```python
from build123d import *

# Parameters (mm, degrees)
F0_W     = 520.7
F0_H     = 457.2
F1_DEPTH = 36.5125
F2_R     = 203.2
F3_R     = 69.85
F4_R     = 22.225
F6_DEPTH = 222.25
F6_TAPER = -1
F8_ANGLE = 180


# Not quite as in the source:
# - a feature names something its author has since deleted; it is built from what else it names


with BuildPart() as f1:
    # F0 (on Top) → F1 (new body)
    with BuildSketch(Plane.XY):
        Rectangle(F0_W, F0_H)
    extrude(amount=F1_DEPTH)

    # F2
    f2_edges = [f1.edges().sort_by_distance(p)[0] for p in [
        (-260.35, -228.6, 18.25625),
        (260.35, -228.6, 18.25625),
    ]]
    fillet(f2_edges, radius=F2_R)

    # F3
    f3_edges = [f1.edges().sort_by_distance(p)[0] for p in [
        (260.35, 228.6, 18.25625),
        (-260.35, 228.6, 18.25625),
    ]]
    fillet(f3_edges, radius=F3_R)

    # F4
    f4_edges = [f1.edges().sort_by_distance(p)[0] for p in [
        (0, 228.6, 36.5125),
    ]]
    fillet(f4_edges, radius=F4_R)

    # F5 (on face) → F6 (cut)
    with BuildSketch(Plane(origin=(0, 228.6, 0), x_dir=(-1, 0, 0), z_dir=(0, 1, 0))):
        with BuildLine():
            Line((0, 181.2540946981), (-105.1541626057, 217.9785540242))
            ThreePointArc((-105.1541626057, 217.9785540242), (-243.9245415433, 129.7884295676), (-126.0241182101, 15.1838646496))
            Line((-126.0241182101, 15.1838646496), (0, 31.7752545682))
            Line((0, 31.7752545682), (126.0241182101, 15.1838646496))
            ThreePointArc((126.0241182101, 15.1838646496), (243.9245415433, 129.7884295676), (105.1541626057, 217.9785540242))
            Line((105.1541626057, 217.9785540242), (0, 181.2540946981))
        make_face()
    extrude(amount=-F6_DEPTH, taper=F6_TAPER, mode=Mode.SUBTRACT)

    # F7 (on face) → F8 (revolve, cut)
    with BuildSketch(Plane(origin=(0, 6.35, 0), x_dir=(-1, 0, 0), z_dir=(0, 1, 0))):
        with BuildLine():
            Line((0, 36.5125), (-210.3489459995, 36.5125))
            ThreePointArc((-210.3489459995, 36.5125), (-170.6122176221, 14.8981545045), (-125.5177564428, 11.3376651729))
            Line((-125.5177564428, 11.3376651729), (0, 27.8623913002))
            Line((0, 27.8623913002), (0, 36.5125))
        make_face()
    revolve(axis=Axis((0, 6.35, 32.1874456501), (0, 0, -1)), revolution_arc=F8_ANGLE, mode=Mode.SUBTRACT)


solid = f1.part
```
Work out the finished part from the listing and answer in its coordinate system (mm). A direction names the side the tool comes from. Round coordinates to 2 decimals unless told otherwise and drop trailing zeros. Return JSON: item names as keys, results as strings. Group by question number.
Q1. Find the intervals of material crossed by L1, parallel to Z at x = -236.5, y = -54.5; L2, parallel to X at y = 156, z = 31.5; L3, parallel to X at y = -129.5, z = 34, in increasing order.
Q2. Each of these flat-tipped pins is pushed along its axis until it touches: pin 1 Ø12 at (y, z) = (149, 23.5) entering from -X; pin 2 Ø4 at (x, z) = (-10.5, 27) entering from -Y; pin 3 Ø6 at (x, z) = (-67, 19.5) entering from -Y. Where does it stop, or does it pass through?
Q3. For faces 5 (the conical face through (170.668, 115.919, 16.912)), 6 (the flat face through (260.35, 65, 7)), determine the directions among +Z, -Z, +X, -X, +Y, -Y from which every point of the face is accessible in a straight line to the end or side of a thin tool.
Q4. The mould has two halves that part along Y. Classify faces 1 (the conical face through (-169.467, 115.919, 16.555)), 2 (the flat face through (-54, -198, 36.512)), 3 (the cylindrical face through (239.345, 208.681, 7.244)), 4 (the cylindrical face through (199.2, -170.7, 7.2)): released by +Y, released by -Y, zero draft, split by the parting line, or undercut.
Solved:
{
 "1": {"L1": "0 to 36.5", "L2": "-252.18 to -199.51, 199.51 to 252.18", "L3": "-217.57 to -156.59, 156.59 to 217.57"},
 "2": {"pin 1": "x = -260.12", "pin 2": "y = -225.85", "pin 3": "y = -228.28"},
 "3": {"face 5": "+Z", "face 6": "+Z, -Z, +X, +Y, -Y"},
 "4": {"face 1": "undercut", "face 2": "zero draft", "face 3": "released by +Y", "face 4": "released by -Y"}
}
